from build123d import *

# Parameters (mm, degrees)
SKETCH_1_R          = 7.5
SKETCH_1_R_2        = 1.25
EXTRUDE_1_DEPTH     = 3
SKETCH_2_R          = 6.5
EXTRUDE_2_DEPTH     = 63
SKETCH_3_R          = 1.25
CUT_EXTRUDE_1_DEPTH = 64.886618317
FILLET_1_R          = 0.5


with BuildPart() as part:
    # Эскиз1 → Бобышка-Вытянуть1 (new body)
    with BuildSketch(Plane(origin=(0, 0, 0), x_dir=(1, 0, 0), z_dir=(0, 1, 0))):
        with Locations(Location((0, 0, 0), (0, 0, 270))):
            Circle(SKETCH_1_R)
        with Locations(Location((0, 0, 0), (0, 0, 270))):
            Circle(SKETCH_1_R_2, mode=Mode.SUBTRACT)
    extrude(amount=EXTRUDE_1_DEPTH)

    # Эскиз2 → Бобышка-Вытянуть2 (add)
    with BuildSketch(Plane(origin=(0, 3, 0), x_dir=(1, 0, 0), z_dir=(0, 1, 0))):
        with Locations(Location((0, 0, 0), (0, 0, 270))):
            Circle(SKETCH_2_R)
    extrude(amount=EXTRUDE_2_DEPTH)

    # Эскиз3 → Вырез-Вытянуть1 (cut, through all)
    with BuildSketch(Plane.XZ.offset(-3)):
        with Locations(Location((0, 0, 0), (0, 0, 270))):
            Circle(SKETCH_3_R)
    extrude(amount=-CUT_EXTRUDE_1_DEPTH, mode=Mode.SUBTRACT)

    # Скругление1
    fillet_1_edges = [part.edges().sort_by_distance(p)[0] for p in [
        (0, 66, -6.5),
        (0, 3, -7.5),
    ]]
    fillet(fillet_1_edges, radius=FILLET_1_R)


solid = part.part
Can you work these out from the model? Positions are in its coordinate system, mm. A direction names the side the tool comes from. Coordinates: 2 decimals unless noted, no trailing zeros. Write each loop counter-clockwise with the first axis right and the second up, starting at its lowest first coordinate (ties: lowest second). Pieces come first, ordered by that corner, then holes. Notation, with made-up numbers: (17, 66.25) -> (21, 66.25) arc R15 ccw to (21, 89.25) -> close; hole circle Ø6 at (-2, 79.25). An arc over 180 degrees is marked (long way). Write each question's results on one line, items separated by ' | '. Start each with the question number.
Item 1: Please list where these lines run through material, in increasing order: probe 1 along X at (y, z) = (36.5, 0); probe 2 along X at (y, z) = (1.55, 0); probe 3 along X at (y, z) = (34, 2.5).
Item 2: I'm going to push flat-ended pins straight in: P1, Ø8, axis at x = 3, z = 4, coming from the -Y side; P2, Ø2, axis at y = 21.5, z = 3.5, coming from the -X side; P3, Ø1.5, axis at x = 2, y = 23.5, coming from the -Z side; P4, Ø2, axis at y = 12.5, z = 4.5, coming from the -X side. Where does each tip first touch, or does it pass through?
Item 3: If we section it at A-A, the plane x = 0: Write out the boundary of the cut face in (y, z).
Item 4: If we section it at C-C, the plane y = 14: Write out the boundary of the cut face in (x, z).
Item 5: On a 3-axis mill with a long thin cutter (end or side, diameter ignored), from which of +Z, -Z, +X, -X, +Y, -Y can I reach the whole of each face in a straight line? I mean faces 1 (the flat face through (0, 0, 2)), 2 (the cylindrical face through (-3.955, 33.812, -5.158)). Say none if no direction works.
Item 6: If we section it at B-B, the plane z = 0: Write out the boundary of the cut face in (x, y).
Answer block:
1) probe 1: -6.5 to -1.25, 1.25 to 6.5 | probe 2: -7.5 to -1.25, 1.25 to 7.5 | probe 3: -6 to 6
2) P1: y = 0 | P2: x = -6 | P3: z = -6.38 | P4: x = -5.48
3) outline: (0, -7.5) -> (2.5, -7.5) arc R0.5 ccw to (3, -7) -> (3, -6.5) -> (65.5, -6.5) arc R0.5 ccw to (66, -6) -> (66, -1.25) -> (0, -1.25) -> close; (0, 1.25) -> (66, 1.25) -> (66, 6) arc R0.5 ccw to (65.5, 6.5) -> (3, 6.5) -> (3, 7) arc R0.5 ccw to (2.5, 7.5) -> (0, 7.5) -> close
4) outline: circle Ø13 at (0, 0); hole circle Ø2.5 at (0, 0)
5) face 1: +Z, -Z, +X, -X, -Y | face 2: +Y
6) outline: (-7.5, 0) -> (-1.25, 0) -> (-1.25, 66) -> (-6, 66) arc R0.5 ccw to (-6.5, 65.5) -> (-6.5, 3) -> (-7, 3) arc R0.5 ccw to (-7.5, 2.5) -> close; (1.25, 0) -> (7.5, 0) -> (7.5, 2.5) arc R0.5 ccw to (7, 3) -> (6.5, 3) -> (6.5, 65.5) arc R0.5 ccw to (6, 66) -> (1.25, 66) -> close
